Build history of the part. All positions in model axes, mm. A direction names the side the tool comes from. Round coordinates to 2 decimals unless told otherwise and drop trailing zeros. Write each loop counter-clockwise with the first axis right and the second up, starting at its lowest first coordinate (ties: lowest second). Pieces come first, ordered by that corner, then holes. Notation, with made-up numbers: M -8.5,53.5 L 41.5,53.5 A9 cw 41.5,64.5 Z; hole C -20.5,80 d3. An arc over 180 degrees is marked long. Use a Markdown table: item, result.
from build123d import *

# Parameters (mm, degrees)
SKETCH1_W           = 79
SKETCH1_H           = 59
BOSS_EXTRUDE1_DEPTH = 5
SKETCH2_R           = 1.5
SKETCH2_W           = 23
SKETCH2_H           = 17.75
CUT_EXTRUDE1_DEPTH  = 2.6
SKETCH3_W           = 33.7
SKETCH3_H           = 35.5
CUT_EXTRUDE2_DEPTH  = 2.4
FILLET1_R           = 4


with BuildPart() as part:
    # Sketch1 → Boss-Extrude1 (new body)
    with BuildSketch(Plane.XY):
        Rectangle(SKETCH1_W, SKETCH1_H)
    extrude(amount=BOSS_EXTRUDE1_DEPTH)

    # Sketch2 → Cut-Extrude1 (cut)
    with BuildSketch(Plane.XY.offset(5)):
        with Locations((-4.15, 15.71)):
            Circle(SKETCH2_R)
        with Locations((-4.15, -15.71)):
            Circle(SKETCH2_R)
        with Locations((-33.85, -15.71)):
            Circle(SKETCH2_R)
        with Locations((-33.85, 15.71)):
            Circle(SKETCH2_R)
        with Locations((-19, -8.875)):
            Rectangle(SKETCH2_W, SKETCH2_H)
        with Locations((-19, 8.875)):
            Rectangle(SKETCH2_W, SKETCH2_H)
    extrude(amount=-CUT_EXTRUDE1_DEPTH, mode=Mode.SUBTRACT)

    # Sketch3 → Cut-Extrude2 (cut)
    with BuildSketch(Plane(origin=(0, 0, 0), x_dir=(-1, 0, 0), z_dir=(0, 0, -1))):
        with Locations((19, 0)):
            Rectangle(SKETCH3_W, SKETCH3_H)
    extrude(amount=-CUT_EXTRUDE2_DEPTH, mode=Mode.SUBTRACT)

    # Fillet1
    fillet1_edges = [part.edges().sort_by_distance(p)[0] for p in [
        (39.5, -29.5, 2.5),
        (-39.5, -29.5, 2.5),
        (-39.5, 29.5, 2.5),
        (39.5, 29.5, 2.5),
    ]]
    fillet(fillet1_edges, radius=FILLET1_R)


solid = part.part
Q1. Two-plate mould, pull along X, no slides. Class faces 1 (the cylindrical face through (-4.345, 17.197, 3.718)), 2 (the cylindrical face through (38.297, -28.359, 2.535)), 3 (the flat face through (0, 29.5, 2)): +X half, -X half, draft (parallel to the pull), parting line (faces both ways), or undercut.
Response values:
| item | result |
|---|---|
| face 1 | undercut |
| face 2 | +X half |
| face 3 | draft |
Q2. Cut at B-B on z = 1.4. Give the cut face in (x, y).
Response values:
| item | result |
|---|---|
| outline | M -39.5,-25.5 A4 ccw -35.5,-29.5 L 35.5,-29.5 A4 ccw 39.5,-25.5 L 39.5,25.5 A4 ccw 35.5,29.5 L -35.5,29.5 A4 ccw -39.5,25.5 Z; hole M -35.85,-17.75 L -2.15,-17.75 L -2.15,17.75 L -35.85,17.75 Z |
Q3. Drop a flat-ended pin along its axis: P1, Ø1.6, axis at x = -33, y = -3.5, coming from the -Z side. Give the stop position or say it passes through.
Response values:
| item | result |
|---|---|
| P1 | stops at z = 2.4 |
Q4. Cut at C-C on x = -33.85. Give the cut face in (y, z).
Response values:
| item | result |
|---|---|
| outline | M -29.5,0 L -17.75,0 L -17.75,2.4 L -17.21,2.4 L -17.21,5 L -29.5,5 Z; M -14.21,2.4 L 14.21,2.4 L 14.21,5 L -14.21,5 Z; M 17.21,2.4 L 17.75,2.4 L 17.75,0 L 29.5,0 L 29.5,5 L 17.21,5 Z |
Q5. Which spindle directions (+Z, -Z, +X, -X, +Y, -Y) get a long thin tool onto all of the face, cutting with end or side? Do faces 4 (the flat face through (-30.5, 0, 4)), 5 (the flat face through (-35.85, 0, 1)), 6 (the cylindrical face through (-38.359, -28.297, 2.535)). Say none if no direction does.
Response values:
| item | result |
|---|---|
| face 4 | +Z, -Z |
| face 5 | -Z |
| face 6 | +Z, -Z, -X, -Y |
Q6. Cut at D-D on x = -9. Give the cut face in (y, z).
Response values:
| item | result |
|---|---|
| outline | M -29.5,0 L -17.75,0 L -17.75,5 L -29.5,5 Z; M 17.75,0 L 29.5,0 L 29.5,5 L 17.75,5 Z |
Q7. Drill centre lines: L1, parallel to Y at x = -33.85, z = 3.15; L2, parallel to Y at x = -24, z = 2.1; L3, parallel to X at y = -13.5, z = 2.9. Where is each one in solid material? Low to high.
Response values:
| item | result |
|---|---|
| L1 | y = -29.5 to -17.21, -14.21 to 14.21, 17.21 to 29.5 |
| L2 | y = -29.5 to -17.75, 17.75 to 29.5 |
| L3 | x = -39.5 to -30.5, -7.5 to 39.5 |
Q8. Cut at A-A on y = 5. Give the cut face in (x, z).
Response values:
| item | result |
|---|---|
| outline | M -39.5,0 L -35.85,0 L -35.85,2.4 L -30.5,2.4 L -30.5,5 L -39.5,5 Z; M -7.5,2.4 L -2.15,2.4 L -2.15,0 L 39.5,0 L 39.5,5 L -7.5,5 Z |
